The figure shows three views and two pictorial views of one solid part (mm, origin at its lowest corner). Answer the questions. A direction names the side the tool comes from. Give positions to 0.01 mm unless a question says otherwise; leave off trailing zeros. Loops run counter-clockwise (first coordinate to the right, second up) from the corner with the lowest first, then second, coordinate; pieces in that order, holes last. Notation, with made-up numbers: (14, 41.25) - (18, 41.25) arc R12 cw to (18, 53.25) - close; hole circle Ø6 at (-15.75, 36). An arc over 180 degrees is marked (long way). Write each question's results on one line, items separated by ' | '.
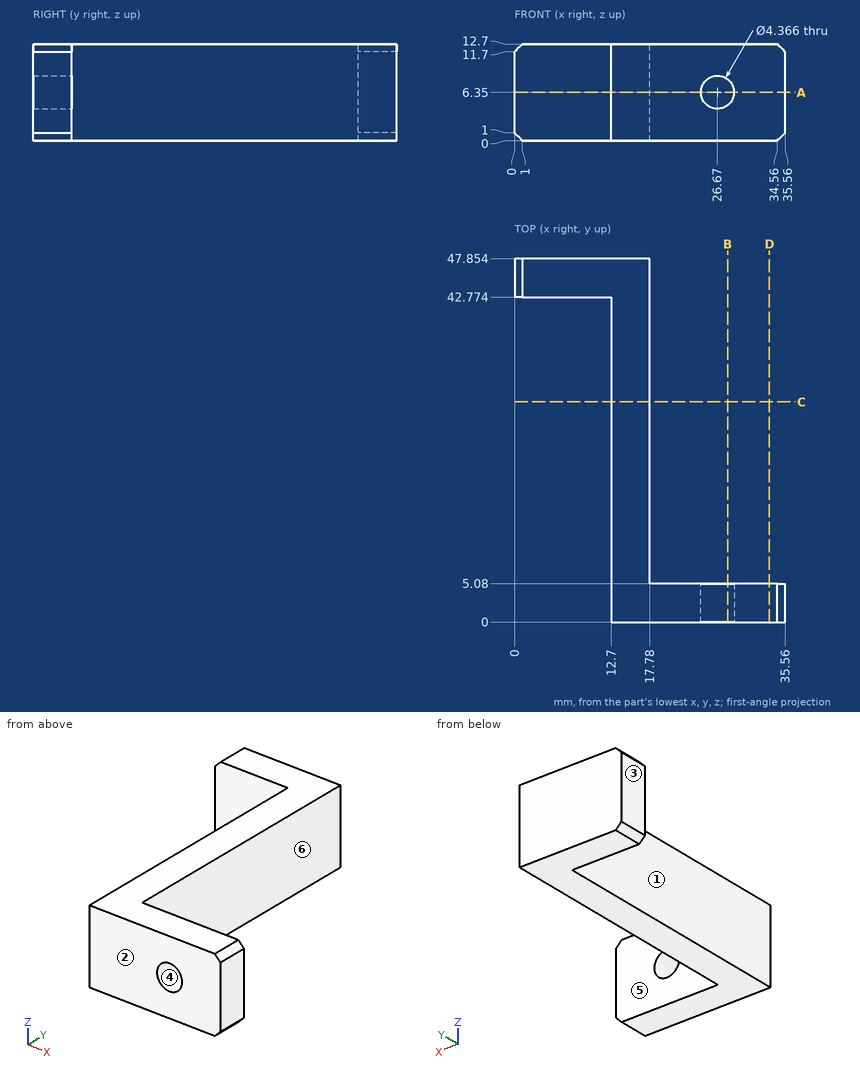
Item 1: Find the intervals of material crossed by line 1 along X through (y, z) = (1.8, 6.35); line 2 along Z through (x, y) = (26.67, 3.8); line 3 along X through (y, z) = (8, 5.25), in increasing order. Write a range as [from, to].
Values found:
line 1: x = [12.7, 24.49], [28.85, 35.56] | line 2: z = [0, 4.17], [8.53, 12.7] | line 3: x = [12.7, 17.78]
Item 2: A cutting plane is placed at B-B, the plane x = 28. Determine the outline of the cut face in (y, z).
Values found:
outline: (0, 0) - (5.08, 0) - (5.08, 4.62) - (0, 4.62) - close; (0, 8.08) - (5.08, 8.08) - (5.08, 12.7) - (0, 12.7) - close
Item 3: For the marked faces 1 and 2, determine the directions among +Z, -Z, +X, -X, +Y, -Y from which every point of the face is accessible in a straight line to the end or side of a thin tool.
Values found:
face 1: +Z, -Z, -X, -Y | face 2: +Z, -Z, +X, -X, -Y
Item 4: Flat-ended cylindrical pins translate along their axes: P1, Ø6.5, axis at x = 26, z = 7.5, coming from the +Y side; P2, Ø1.5, axis at y = 38, z = 4, coming from the -X side; P3, Ø3.5, axis at x = 26.67, z = 6.35, coming from the -Y side. Find the tip coordinate at first contact, or state that the pin passes through.
Values found:
P1: stops at y = 5.08 | P2: stops at x = 12.7 | P3: passes through
Item 5: A cutting plane is placed at A-A, the plane z = 6.35. Determine the outline of the cut face in (x, y), plus the area to 3 significant figures.
Values found:
outline: (0, 42.77) - (12.7, 42.77) - (12.7, 0) - (24.49, 0) - (24.49, 5.08) - (17.78, 5.08) - (17.78, 47.85) - (0, 47.85) - close; (28.85, 0) - (35.56, 0) - (35.56, 5.08) - (28.85, 5.08) - close | area: 376 mm²
Item 6: A cutting plane is placed at C-C, the plane y = 29. Determine the outline of the cut face in (x, z), plus the area to 3 significant figures.
Values found:
outline: (12.7, 0) - (17.78, 0) - (17.78, 12.7) - (12.7, 12.7) - close | area: 64.5 mm²
Item 7: For a pull along X with two mould halves and no side action, classify the marked faces 3, 4, 5 and 6 as released by +X, released by -X, zero draft, split by the parting line, or undercut.
Values found:
face 3: released by -X | face 4: undercut | face 5: zero draft | face 6: released by +X
Item 8: A cutting plane is placed at D-D, the plane x = 33.5. Determine the outline of the cut face in (y, z).
Values found:
outline: (0, 0) - (5.08, 0) - (5.08, 12.7) - (0, 12.7) - close
